Autodesk Inventor part; units mm, degrees
ref_plane "Work Plane1" through (24, 0, 0) normal (1, 0, 0) x (0, 1, 0)
ref_plane "XZ Plane" through (0, 0, 0) normal (0, 1, 0) x (-1, 0, 0)
ref_plane "XY Plane" through (0, 0, 0) normal (0, 0, 1) x (1, 0, 0)
sketch "Sketch1" plane through (0, 0, 0) normal (0, 0, 1) x (1, 0, 0)
  circle A0 centre (0, 0) radius 5
  dimension "d0" = 10
extrude "Extrusion1" add sketch "Sketch1" along normal blind 7
sketch "Sketch2" plane through (0, 0, 0) normal (1, 0, 0) x (0, 1, 0)
  line L0 (-2.5, 7) -> (2.5, 7)
  line L1 (2.5, 7) -> (2.5, 0)
  line L2 (2.5, 0) -> (-2.5, 0)
  line L3 (-2.5, 0) -> (-2.5, 7)
  line L4 (-2.5, 7) -> (2.5, 0) construction
  line L5 (2.5, 7) -> (-2.5, 0) construction
  line L6 (-5, 0) -> (5, 0)
  point P0 (0, 0)
  point P1 (0, 3.5)
  dimension "d3" = 3.5
  dimension "d4" = 0
  dimension "d5" = 7
  dimension "d6" = 5
sketch "Sketch3" plane through (0, 0, 0) normal (0, 1, 0) x (-1, 0, 0)
  arc A0 (-25, 22.5) -> (-5, 2.5) centre (-5, 22.5) ccw
  line L0 (-5, 2.5) -> (0, 2.5)
  line L1 (-25, 22.5) -> (-25, 27.5)
  point P0 (0, 0)
  dimension "d14" = 2.5
  dimension "d15" = 5
  dimension "d17" = 5
  dimension "d24" = 5
  dimension "d55" = 20
  dimension "d56" = 0
  dimension "d57" = 20
sweep "Sweep1" add profiles "Sketch2" path "Sketch3"
ref_plane "Work Plane1" through (24, 0, 0) normal (1, 0, 0) x (0, 1, 0)
sketch "Sketch4" plane through (24, 0, 0) normal (1, 0, 0) x (0, 1, 0)
  circle A0 centre (0, 27.5) radius 5
  point P0 (0, 0)
  dimension "d27" = 10
  dimension "d28" = 27.5
  dimension "d29" = 0
extrude "Extrusion2" add sketch "Sketch4" along normal mid plane 7
sketch "Sketch6" plane through (27.5, -2.5, 22.5) normal (-1, 0, 0) x (0, 0, 1)
  circle A0 centre (5, 2.5) radius 3.5
  point P0 (-22.5, 2.5)
  dimension "d32" = 7
  dimension "d33" = 27.5
  dimension "d34" = 0
extrude "Extrusion4" cut sketch "Sketch6" along normal blind 3
sketch "Sketch7" plane through (24.5, 0, 27.5) normal (-1, 0, 0) x (0, 0, 1)
  circle A0 centre (0, 0) radius 2.5
  line L0 (-27.5, 5) -> (-27.5, -5)
  point P0 (-27.5, 0)
  point P1 (-27.5, -2.5)
  point P2 (-27.5, 2.5)
  dimension "d37" = 5
  dimension "d38" = 27.5
  dimension "d39" = 0
extrude "Extrusion5" cut sketch "Sketch7" along normal up to next
sketch "Sketch8" plane through (0, 0, 0) normal (0, 0, -1) x (-1, 0, 0)
  circle A0 centre (0, 0) radius 3.5
  dimension "d42" = 7
extrude "Extrusion6" cut sketch "Sketch8" against normal blind 3
sketch "Sketch9" plane through (0, 0, 3) normal (0, 0, -1) x (-1, 0, 0)
  circle A0 centre (0, 0) radius 2.5
  dimension "d45" = 5
extrude "Extrusion7" cut sketch "Sketch9" against normal up to next
fillet "Fillet1" radius 5 4 edges at (24, -2.5, 23.1699) (24, 2.5, 23.1699) (4.3301, -2.5, 3.5) (4.3301, 2.5, 3.5)
sketch "Sketch10" plane through (20.5, 0, 27.5) normal (-1, 0, 0) x (0, 0, 1)
  circle A0 centre (0, 0) radius 3.5
  circle A1 centre (0, 0) radius 2.5
  point P0 (-27.5, 0)
  dimension "d49" = 7
extrude "Extrusion8" cut sketch "Sketch10" against normal blind 3
sketch "Sketch11" plane through (0, 0, 7) normal (0, 0, 1) x (1, 0, 0)
  circle A0 centre (0, 0) radius 3.5
  circle A1 centre (0, 0) radius 2.5
  dimension "d52" = 7
extrude "Extrusion9" cut sketch "Sketch11" against normal blind 3
equation "\"d55\" = width"
equation "\"d57\" = height"
equation "\"d38\" = d28"
properties part number "Link"
Here's how the part is built. I have some questions about the finished solid (model axes, mm). A direction names the side the tool comes from. Round coordinates to 2 decimals unless told otherwise and drop trailing zeros. Write each loop counter-clockwise with the first axis right and the second up, starting at its lowest first coordinate (ties: lowest second). Pieces come first, ordered by that corner, then holes.
Q1. If we section it at B-B on y = 0: Give the number of separate pieces and of enclosed holes in the cut face, plus the area to 3 significant figures.
Q2. Will these pins go through, and if not, where does the flat tip stop? P1, Ø5, axis at x = -2, y = 1.5, coming from the +Z side; P2, Ø2, axis at y = -0.5, z = 26.5, coming from the -X side; P3, Ø3, axis at x = 11, y = -2, coming from the -Z side; P4, Ø16.5, axis at x = 13.5, z = 14.5, coming from the -Y side.
Q3. If we section it at A-A on z = 27.5: Write out the boundary of the cut face in (x, y), plus the area to 3 significant figures.
Q4. If we mould it in two halves opening along Y, with no side actions, what happens to faces 4 (the flat face through (3.3, -2.2, 7)), 5 (the flat face through (17, 2.5, 10)), 6 (the flat face through (23.5, 1, 25)), 7 (the cylindrical face through (0.54, -2.44, 3.49))? For each: +Y half, -Y half, draft (parallel to the pull), parting line (faces both ways), or undercut.
Q5. If we section it at D-D on z = 4.5: Write out the boundary of the cut face in (x, y), plus the area to 3 significant figures.
Q6. Please list where these lines run through material, in increasing order: probe 1 along Y at (x, z) = (24.25, 27.5); probe 2 along Y at (x, z) = (26.3, 27.5); probe 3 along Y at (x, z) = (10, 4.5).
Q7. If we section it at C-C on x = 0: Write out the boundary of the cut face in (y, z), plus the area to 3 significant figures.
Q8. Which directions (+Z, -Z, +X, -X, +Y, -Y) give clear straight access to the entire face, cutting with the end or side of a thin tool? Please do faces 1 (the flat face through (17, -2.5, 11)), 2 (the flat face through (2, -2, 4)), 3 (the cylindrical face through (21.98, 1.05, 30.84)).
Answer below:
1. separate pieces: 3
1. enclosed holes: 0
1. area: 255 mm2
2. P1: stops at z = 7
2. P2: passes through
2. P3: stops at z = 0.45
2. P4: stops at y = -2.5
3. outline: (20.5, -5) - (27.5, -5) - (27.5, -3.5) - (24.5, -3.5) - (24.5, -2.5) - (23.5, -2.5) - (23.5, -3.5) - (20.5, -3.5) - close; (20.5, 3.5) - (23.5, 3.5) - (23.5, 2.5) - (24.5, 2.5) - (24.5, 3.5) - (27.5, 3.5) - (27.5, 5) - (20.5, 5) - close
3. area: 23.0 mm2
4. face 4: draft
4. face 5: +Y half
4. face 6: undercut
4. face 7: undercut
5. outline: (3.31, -3.75) arc R5 cw to (6.61, -2.5) - (18.5, -2.5) - (18.5, 2.5) - (6.61, 2.5) arc R5 cw to (3.31, 3.75) arc R5 ccw (long way) to start; hole circle Ø7 at (0, 0)
5. area: 110 mm2
6. probe 1: y = -5 to -2.5, 2.5 to 5
6. probe 2: y = -5 to -3.5, 3.5 to 5
6. probe 3: y = -2.5 to 2.5
7. outline: (-5, 0) - (-3.5, 0) - (-3.5, 3) - (-2.5, 3) - (-2.5, 4) - (-3.5, 4) - (-3.5, 7) - (-5, 7) - close; (2.5, 3) - (3.5, 3) - (3.5, 0) - (5, 0) - (5, 7) - (3.5, 7) - (3.5, 4) - (2.5, 4) - close
7. area: 23.0 mm2
8. face 1: -Z, +X, -Y
8. face 2: +Z
8. face 3: -X
